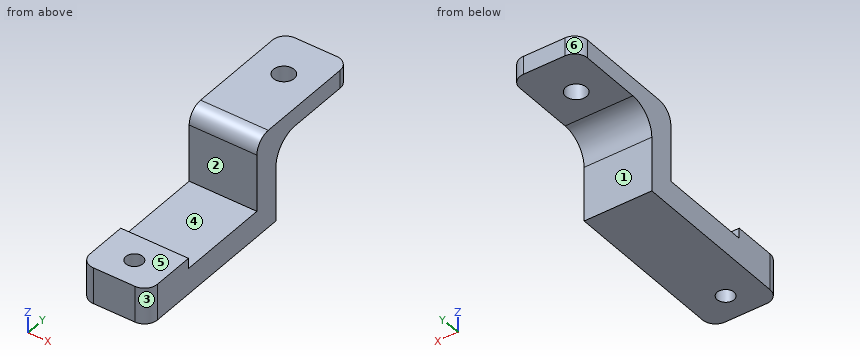
```python
from build123d import *

# Parameters (mm, degrees)
F1_DEPTH = 13
F2_R     = 1.625
F3_DEPTH = 25
F4_R     = 2
F5_DEPTH = 25
F6_R     = 5
F7_R     = 3
F8_R     = 2.5


with BuildPart() as f1:
    # F0 (on Right) → F1 (new body)
    with BuildSketch(Plane.YZ):
        Polygon((10.648379, 0), (0, 0), (0, -7), (33.648379, -7), (33.648379, 8.5), (53.068466, 8.5), (53.068466, 12), (28.648379, 12), (28.648379, -2), (10.648379, -2), align=None)
    extrude(amount=F1_DEPTH)

    # F2 (on face) → F3 (cut)
    with BuildSketch(Plane.XY):
        with Locations((6.5, 5.32419)):
            Circle(F2_R)
    extrude(amount=-F3_DEPTH, mode=Mode.SUBTRACT)

    # F4 (on face) → F5 (cut)
    with BuildSketch(Plane.XY.offset(12)):
        with Locations((6.5, 44.636294)):
            Circle(F4_R)
    extrude(amount=-F5_DEPTH, mode=Mode.SUBTRACT)

    # F6
    f6_edges = [f1.edges().sort_by_distance(p)[0] for p in [
        (6.5, 33.648379, 8.5),
    ]]
    fillet(f6_edges, radius=F6_R)

    # F7
    f7_edges = [f1.edges().sort_by_distance(p)[0] for p in [
        (6.5, 28.648379, 12),
    ]]
    fillet(f7_edges, radius=F7_R)

    # F8
    f8_edges = [f1.edges().sort_by_distance(p)[0] for p in [
        (13, 53.068466, 10.25),
        (0, 53.068466, 10.25),
        (13, 0, -3.5),
        (0, 0, -3.5),
    ]]
    fillet(f8_edges, radius=F8_R)


solid = f1.part
```
The listing builds one solid part. Answer for the finished solid, in the listing's coordinates (mm). Face numbers are marked on the shaded views. A direction names the side the tool comes from. Coordinates: 2 decimals unless noted, no trailing zeros. Write each loop counter-clockwise with the first axis right and the second up, starting at its lowest first coordinate (ties: lowest second). Pieces come first, ordered by that corner, then holes. Notation, with made-up numbers: M 13.25,36 L 22.25,36 A22 cw 22.25,43 Z; hole C 67,12 d2. An arc over 180 degrees is marked long. Use a Markdown table: item, result. Add a question column.
1. Section D-D (z = -4.5) is taken. Give the vertices of the cut face in (x, y) (3 decimals).
2. Given P1, Ø6, axis at x = 4, y = 7.5, coming from the +Z side; P2, Ø3, axis at x = 2, z = 2, coming from the +Y side; P3, Ø6.5, axis at x = 6.5, y = 43.5, coming from the -Z side; P4, Ø5, axis at y = 36, z = -5, coming from the +X side, each flat-ended and moving along its own axis, determine where each tip first touches the part or whether it passes through.
3. Which of the six approach directions +Z, -Z, +X, -X, +Y, -Y give full straight-line access (tool end or side, diameter ignored) to the marked faces 1, 2 and 3?
4. Section B-B (z = -1.5) is taken. Give the vertices of the cut face in (x, y) (3 decimals), plus the area to 3 significant figures.
5. Straight lines are drawn through the part: line 1 along Y through (x, z) = (6.5, -3); line 2 along Y through (x, z) = (6.5, -1.5); line 3 along Z through (x, y) = (11.5, 7). For each, find the intervals that lie inside material, in ascending order. Write a range as [from, to].
6. For a pull along Y with two mould halves and no side action, classify the marked faces 4, 5 and 6 as +Y half, -Y half, draft (parallel to the pull), parting line (faces both ways), or undercut.
7. Section A-A (x = 6.5) is taken. Give the vertices of the cut face in (y, z).
8. Section C-C (x = 3) is taken. Give the vertices of the cut face in (y, z), plus the area to 3 significant figures.
Data:
| question | item | result |
|---|---|---|
| 1 | outline | M 0,2.5 A2.5 ccw 2.5,0 L 10.5,0 A2.5 ccw 13,2.5 L 13,33.648 L 0,33.648 Z; hole C 6.5,5.324 d3.25 |
| 2 | P1 | stops at z = 0 |
| 2 | P2 | stops at y = 33.65 |
| 2 | P3 | stops at z = 8.5 |
| 2 | P4 | stops at x = 13 |
| 3 | face 1 | -Z, +X, -X, +Y |
| 3 | face 2 | +Z, +X, -X |
| 3 | face 3 | +Z, -Z, +X, -Y |
| 4 | outline | M 0,2.5 A2.5 ccw 2.5,0 L 10.5,0 A2.5 ccw 13,2.5 L 13,10.648 L 0,10.648 Z; M 0,28.648 L 13,28.648 L 13,33.648 L 0,33.648 Z; hole C 6.5,5.324 d3.25 |
| 4 | area | 192 mm2 |
| 5 | line 1 | y = [0, 3.7], [6.95, 33.65] |
| 5 | line 2 | y = [0, 3.7], [6.95, 10.65], [28.65, 33.65] |
| 5 | line 3 | z = [-7, 0] |
| 6 | face 4 | undercut |
| 6 | face 5 | draft |
| 6 | face 6 | +Y half |
| 7 | outline | M 0,-7 L 3.7,-7 L 3.7,0 L 0,0 Z; M 6.95,-7 L 33.65,-7 L 33.65,3.5 A5 cw 38.65,8.5 L 42.64,8.5 L 42.64,12 L 31.65,12 A3 ccw 28.65,9 L 28.65,-2 L 10.65,-2 L 10.65,0 L 6.95,0 Z; M 46.64,8.5 L 53.07,8.5 L 53.07,12 L 46.64,12 Z |
| 8 | outline | M 0,-7 L 33.65,-7 L 33.65,3.5 A5 cw 38.65,8.5 L 53.07,8.5 L 53.07,12 L 31.65,12 A3 ccw 28.65,9 L 28.65,-2 L 10.65,-2 L 10.65,0 L 0,0 Z |
| 8 | area | 331 mm2 |
